Geometry check sheet. Reference: the model listing, model coordinates, mm. Coordinates: 2 decimals unless noted, no trailing zeros. Write each loop counter-clockwise with the first axis right and the second up, starting at its lowest first coordinate (ties: lowest second). Pieces come first, ordered by that corner, then holes. Notation, with made-up numbers: M 86,67 L 116,67 A25 cw 116,106 Z; hole C -6.5,-11.5 d10. An arc over 180 degrees is marked long. Put each result on its own line as item: value. Start each with the question number.
1) Mould release check, pull along Y, two halves, no side actions. Record for faces 1 (the flat face through (1, -1.27, 1)), 2 (the flat face through (1, 13, 2.54)), 3 (the flat face through (2.54, 6, 1)), 4 (the flat face through (0, 6, 1)): released by +Y, released by -Y, zero draft, split by the parting line, or undercut.
2) Cross-section at B-B on z = 0.3. Record the cut outline in (x, y), plus the area to 3 significant figures.
3) Cross-section at A-A on x = 6.25. Record the cut outline in (y, z).
4) Scan lines: line 1 along Y through (x, z) = (7, 1.1); line 2 along Y through (x, z) = (2, 0.2); line 3 along X through (y, z) = (11.25, 0.55). Record each from-to range of solid material in increasing order.
5) Gauge pin test, flat ends, axial feed: pin 1 (0.5 mm diameter, centred on x = 5, z = 1.5, fed in from +Y); pin 2 (0.7 mm diameter, centred on x = 6.5, z = 1, fed in from -Y); pin 3 (3 mm diameter, centred on x = 6.5, y = 5, fed in from -Z); pin 4 (6 mm diameter, centred on x = 1.5, y = 2, fed in from -Z). Record the tip position at first contact, or that the pin passes through.
6) Cross-section at C-C on y = 2.5. Record the cut outline in (x, z), plus the area to 3 significant figures.
from build123d import *

# Parameters (mm, degrees)
PLASTIC_DEPTH   = 2.54
SKETCH2_W       = 11.44
SKETCH2_H       = 0.6
CONTACT_DEPTH   = 0.3
CHAMFER1_SIZE   = 0.1
LPATTERN1_COUNT = 6
LPATTERN1_PITCH = 2.54


with BuildPart() as part:
    # Sketch1 → Plastic (new body)
    with BuildSketch(Plane(origin=(0, 0, 0), x_dir=(0, 0, -1), z_dir=(1, 0, 0))):
        Polygon((-2.04, 1.27), (-0.5, 1.27), (0, 0.77), (0, -0.77), (-0.5, -1.27), (-2.04, -1.27), (-2.54, -0.77), (-2.54, 0.77), align=None)
    extrude(amount=PLASTIC_DEPTH)

    # Sketch2 → Contact (add, symmetric)
    with BuildSketch(Plane(origin=(0, 0, 0), x_dir=(1, 0, 0), z_dir=(0, 1, 0))):
        with Locations((3.18, -1.27)):
            Rectangle(SKETCH2_W, SKETCH2_H)
    extrude(amount=CONTACT_DEPTH, both=True)

    # Chamfer1
    chamfer1_edges = [part.edges().sort_by_distance(p)[0] for p in [
        (8.9, 0, 0.97),
        (8.9, 0.3, 1.27),
        (-2.54, 0, 1.57),
        (8.9, -0.3, 1.27),
        (8.9, 0, 1.57),
        (-2.54, -0.3, 1.27),
        (-2.54, 0, 0.97),
        (-2.54, 0.3, 1.27),
    ]]
    chamfer(chamfer1_edges, length=CHAMFER1_SIZE)

    # LPattern1: part ×6


with BuildPart() as part_1:
    add(part.part)
    with Locations(*[(0, i * LPATTERN1_PITCH, 0) for i in range(1, LPATTERN1_COUNT)]):
        add(part.part)


solid = part_1.part
Answer key:
1. face 1: released by -Y
1. face 2: zero draft
1. face 3: undercut
1. face 4: undercut
2. outline: M 0,-1.07 L 2.54,-1.07 L 2.54,1.07 L 0,1.07 Z; M 0,1.47 L 2.54,1.47 L 2.54,3.61 L 0,3.61 Z; M 0,4.01 L 2.54,4.01 L 2.54,6.15 L 0,6.15 Z; M 0,6.55 L 2.54,6.55 L 2.54,8.69 L 0,8.69 Z; M 0,9.09 L 2.54,9.09 L 2.54,11.23 L 0,11.23 Z; M 0,11.63 L 2.54,11.63 L 2.54,13.77 L 0,13.77 Z
2. area: 32.6 mm²
3. outline: M -0.3,0.97 L 0.3,0.97 L 0.3,1.57 L -0.3,1.57 Z; M 2.24,0.97 L 2.84,0.97 L 2.84,1.57 L 2.24,1.57 Z; M 4.78,0.97 L 5.38,0.97 L 5.38,1.57 L 4.78,1.57 Z; M 7.32,0.97 L 7.92,0.97 L 7.92,1.57 L 7.32,1.57 Z; M 9.86,0.97 L 10.46,0.97 L 10.46,1.57 L 9.86,1.57 Z; M 12.4,0.97 L 13,0.97 L 13,1.57 L 12.4,1.57 Z
4. line 1: y = -0.3 to 0.3, 2.24 to 2.84, 4.78 to 5.38, 7.32 to 7.92, 9.86 to 10.46, 12.4 to 13
4. line 2: y = -0.97 to 0.97, 1.57 to 3.51, 4.11 to 6.05, 6.65 to 8.59, 9.19 to 11.13, 11.73 to 13.67
4. line 3: x = 0 to 2.54
5. pin 1: stops at y = 13
5. pin 2: stops at y = -0.3
5. pin 3: stops at z = 0.97
5. pin 4: stops at z = 0
6. outline: M -2.54,1.07 L -2.44,0.97 L 0,0.97 L 0,0 L 2.54,0 L 2.54,0.97 L 8.8,0.97 L 8.9,1.07 L 8.9,1.47 L 8.8,1.57 L 2.54,1.57 L 2.54,2.54 L 0,2.54 L 0,1.57 L -2.44,1.57 L -2.54,1.47 Z
6. area: 11.8 mm²
